For this review, take the finished solid that the model builds, in its own axes (mm). Face numbers are marked on the shaded views. A direction names the side the tool comes from. Give positions to 0.01 mm unless a question says otherwise; leave off trailing zeros. Write each loop counter-clockwise with the first axis right and the second up, starting at its lowest first coordinate (ties: lowest second). Pieces come first, ordered by that corner, then holes.
1) We need section B-B on x = -3.5. Give the boundary of the cut face in (y, z) (1 decimal), and give its area (3 significant figures).
2) Machinability: for the marked faces 1 and 2, which of the approach directions +Z, -Z, +X, -X, +Y, -Y give a long, thin tool a straight path to every point of the face, cutting with its end or side? Answer none if there is none.
3) For P1, Ø3.5, axis at y = 0, z = 11.37, coming from the +X side (3 decimals); P2, Ø3, axis at x = -3.5, z = 5.5, coming from the -Y side; P3, Ø3, axis at x = -6, z = 10.5, coming from the -Y side, all flat-tipped, find the tip position at first contact; note any pin that passes through.
4) We need section A-A on y = 0. Give the boundary of the cut face in (x, z) (3 decimals).
5) We need section C-C on y = 2.5. Give the boundary of the cut face in (x, z) (3 decimals).
6) We need section D-D on z = 6.5. Give the boundary of the cut face in (x, y) (3 decimals).
7) Wall thickness on line 1 along Z through (x, y) = (1.85, 0) (3 decimals); line 2 along Z through (x, y) = (3.5, -7) (3 decimals); line 3 along Z through (x, y) = (-1.5, -0.25) (3 decimals): over which ranges is each line inside the solid? List them lowest first.
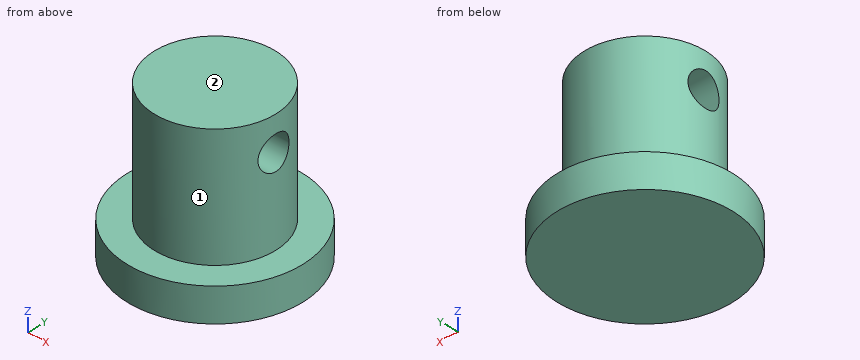
from build123d import *

# Parameters (mm, degrees)
F0_R          = 8.255
F1_DEPTH      = 3.175
F2_R          = 5.715
F3_DEPTH      = 11.43
F4_R          = 1.5875
F5_DEPTH      = 8.256
F5_DEPTH_BACK = 25.4


with BuildPart() as f1:
    # F0 (on Top) → F1 (new body)
    with BuildSketch(Plane.XY):
        Circle(F0_R)
    extrude(amount=F1_DEPTH)

    # F2 (on face) → F3 (join)
    with BuildSketch(Plane.XY.offset(3.175)):
        Circle(F2_R)
    extrude(amount=F3_DEPTH)

    # F4 (on Right) → F5 (cut, two sides)
    with BuildSketch(Plane.YZ) as f5_sk:
        with Locations((0, 11.3665)):
            Circle(F4_R)
    extrude(amount=-F5_DEPTH, mode=Mode.SUBTRACT)
    extrude(f5_sk.sketch, amount=F5_DEPTH_BACK, mode=Mode.SUBTRACT)


solid = f1.part
Results list:
1. outline: (-7.5, 0) - (7.5, 0) - (7.5, 3.2) - (4.5, 3.2) - (4.5, 14.6) - (-4.5, 14.6) - (-4.5, 3.2) - (-7.5, 3.2) - close; hole circle Ø3.2 at (0, 11.4)
1. area: 143 mm2
2. face 1: +Z
2. face 2: +Z, +X, -X, +Y, -Y
3. P1: stops at x = 5.715
3. P2: stops at y = -5.35
3. P3: stops at y = -3.52
4. outline: (-8.255, 0) - (8.255, 0) - (8.255, 3.175) - (5.715, 3.175) - (5.715, 9.779) - (-5.715, 9.779) - (-5.715, 3.175) - (-8.255, 3.175) - close; (-5.715, 12.954) - (5.715, 12.954) - (5.715, 14.605) - (-5.715, 14.605) - close
5. outline: (-7.867, 0) - (7.867, 0) - (7.867, 3.175) - (5.139, 3.175) - (5.139, 14.605) - (-5.139, 14.605) - (-5.139, 3.175) - (-7.867, 3.175) - close
6. outline: circle Ø11.43 at (0, 0)
7. line 1: z = 0 to 9.779, 12.954 to 14.605
7. line 2: z = 0 to 3.175
7. line 3: z = 0 to 9.799, 12.934 to 14.605
